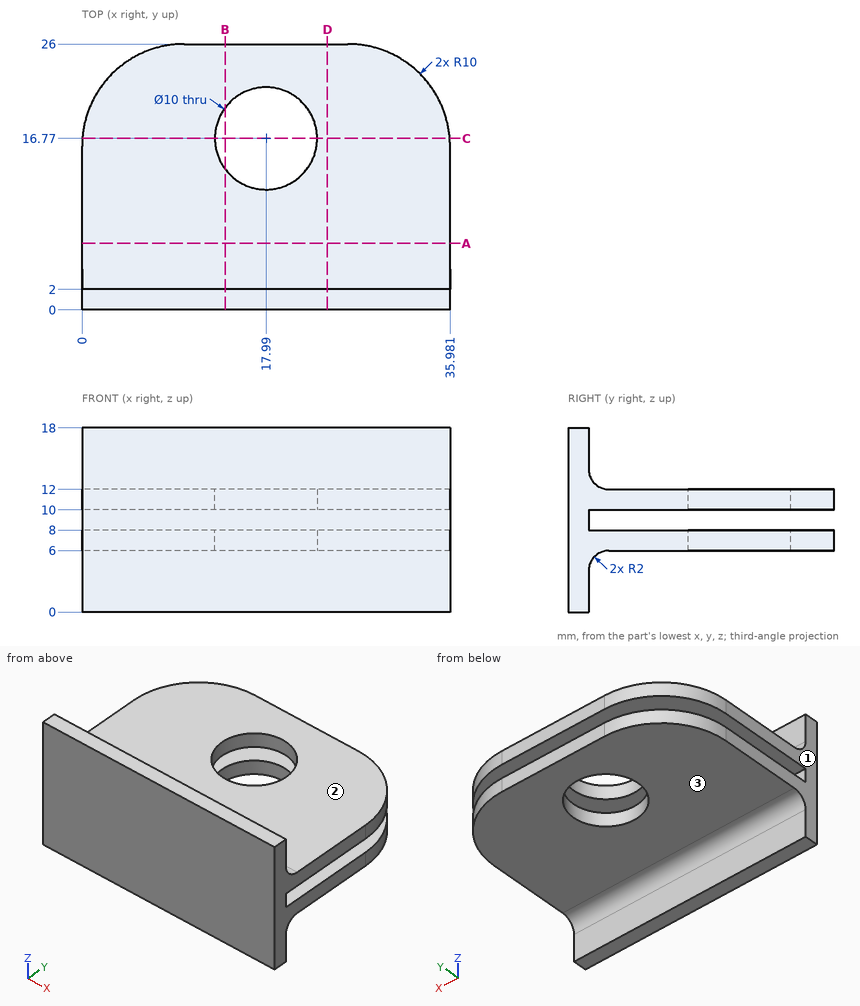
Study the drawing (mm; zero at the part's minimum x, y, z) and answer. A direction names the side the tool comes from. Give positions to 0.01 mm unless a question says otherwise; leave off trailing zeros. Order: outer loops, then holes, each group sorted by start corner. A loop starts at its lowest first (then second) coordinate and runs counter-clockwise, first axis right, second up.
1. Section A-A, the plane y = 6.5 is taken. Determine the outline of the cut face in (x, z), and give its area (3 significant figures).
Result sheet:
outline: (0, 6) - (35.98, 6) - (35.98, 8) - (0, 8) - close; (0, 10) - (35.98, 10) - (35.98, 12) - (0, 12) - close
area: 144 mm2
2. Section D-D, the plane x = 24 is taken. Determine the outline of the cut face in (y, z).
Result sheet:
outline: (0, 0) - (2, 0) - (2, 4) arc R2 cw to (4, 6) - (26, 6) - (26, 8) - (2, 8) - (2, 10) - (26, 10) - (26, 12) - (4, 12) arc R2 cw to (2, 14) - (2, 18) - (0, 18) - close
3. Section C-C, the plane y = 16.77 is taken. Determine the outline of the cut face in (x, z), and give its area (3 significant figures).
Result sheet:
outline: (0.03, 6) - (12.99, 6) - (12.99, 8) - (0.03, 8) - close; (0.03, 10) - (12.99, 10) - (12.99, 12) - (0.03, 12) - close; (22.99, 6) - (35.95, 6) - (35.95, 8) - (22.99, 8) - close; (22.99, 10) - (35.95, 10) - (35.95, 12) - (22.99, 12) - close
area: 104 mm2
4. For the marked faces 1, 2 and 3, determine the directions among +Z, -Z, +X, -X, +Y, -Y from which every point of the face is accessible in a straight line to the end or side of a thin tool.
Result sheet:
face 1: +Z, -Z, -X, +Y, -Y
face 2: +Z, +X, -X, +Y
face 3: -Z, +X, -X, +Y
5. Straight lines are drawn through the part: L1, parallel to Z at x = 24, y = 13.25; L2, parallel to Y at x = 14, z = 16.25; L3, parallel to X at y = 15.5, z = 10.75 (1 decimal). For each, find the intervals that lie inside material, in ascending order.
Result sheet:
L1: z = 6 to 8, 10 to 12
L2: y = 0 to 2
L3: x = 0 to 13.2, 22.8 to 36
6. Section B-B, the plane x = 14 is taken. Determine the outline of the cut face in (y, z).
Result sheet:
outline: (0, 0) - (2, 0) - (2, 4) arc R2 cw to (4, 6) - (13.76, 6) - (13.76, 8) - (2, 8) - (2, 10) - (13.76, 10) - (13.76, 12) - (4, 12) arc R2 cw to (2, 14) - (2, 18) - (0, 18) - close; (19.78, 6) - (26, 6) - (26, 8) - (19.78, 8) - close; (19.78, 10) - (26, 10) - (26, 12) - (19.78, 12) - close
7. Each of these flat-tipped pins is pushed along its axis until it touches: P1, Ø9, axis at x = 17.99, y = 16.77, coming from the -Z side; P2, Ø0.6, axis at x = 15, z = 9.5, coming from the +Y side; P3, Ø4, axis at x = 25, y = 21, coming from the -Z side; P4, Ø12, axis at x = 4.5, y = 18.5, coming from the +Z side. Where does it stop, or does it pass through?
Result sheet:
P1: passes through
P2: stops at y = 2
P3: stops at z = 6
P4: stops at z = 12
